Read the model definition and answer for the solid it produces. Units are mm, in the model's axes. Coordinates: 2 decimals unless noted, no trailing zeros. Write each loop counter-clockwise with the first axis right and the second up, starting at its lowest first coordinate (ties: lowest second). Pieces come first, ordered by that corner, then holes.
1) Find the intervals of material crossed by line 1 (Y direction, x = -254.5, z = 0.25); line 2 (Y direction, x = -270, z = 2.5); line 3 (Y direction, x = -81, z = -2), in increasing order.
2) The part is cut by section A-A (y = -1.5). Determine the outline of the cut face in (x, z), then the cut area to 3 significant figures.
3) Each of these flat-tipped pins is pushed along its axis until it touches: pin 1 Ø1.5 at (x, z) = (-178.5, 1) entering from +Y; pin 2 Ø5 at (x, y) = (-289, 0) entering from +Z; pin 3 Ø7.5 at (x, y) = (-275, 14.5) entering from +Z. Where does it stop, or does it pass through?
from build123d import *

# Parameters (mm, degrees)
BOSS_EXTRUDE1_DEPTH = 500.126
SKETCH2_W           = 12.7
SKETCH2_H           = 24.13
CUT_EXTRUDE1_DEPTH  = 505.455221633
SKETCH3_W           = 487.426
SKETCH3_H           = 14.75620072
BOSS_EXTRUDE2_DEPTH = 3.55599999
SKETCH4_W           = 3.55599999
SKETCH4_H           = 13.202768596
CUT_EXTRUDE2_DEPTH  = 501.46835993
DRAFT1_ANGLE        = 25
DRAFT2_ANGLE        = 25
FILLET1_R           = 0.76200009
FILLET2_R           = 1.98120009
FILLET3_R           = 2.54


with BuildPart() as part:
    # Sketch1 → Boss-Extrude1 (new body)
    with BuildSketch(Plane(origin=(-3.937, 0, 0), x_dir=(0, 0, -1), z_dir=(1, 0, 0))):
        with BuildLine():
            Line((2.311399989, 16.37657286), (2.311399989, -16.37657286))
            ThreePointArc((2.311399989, -16.37657286), (0.354826715, -15.481038557), (-1.770730805, -15.815950332))
            ThreePointArc((-1.770730805, -15.815950332), (-3.400639082, -15.955235788), (-4.710462095, -14.975253591))
            Line((-4.710462095, -14.975253591), (-5.7404, -15.627692517))
            ThreePointArc((-5.7404, -15.627692517), (-3.73586423, -17.127444277), (-1.241474216, -16.914283663))
            ThreePointArc((-1.241474216, -16.914283663), (0.188944014, -16.688900954), (1.505642365, -17.291560998))
            ThreePointArc((1.505642365, -17.291560998), (2.81343034, -17.487614789), (3.53059999, -16.37657286))
            Line((3.53059999, -16.37657286), (3.53059999, 16.37657286))
            ThreePointArc((3.53059999, 16.37657286), (2.81343034, 17.487614789), (1.505642365, 17.291560998))
            ThreePointArc((1.505642365, 17.291560998), (0.188944014, 16.688900954), (-1.241474216, 16.914283663))
            ThreePointArc((-1.241474216, 16.914283663), (-3.73586423, 17.127444277), (-5.7404, 15.627692517))
            Line((-5.7404, 15.627692517), (-4.710462095, 14.975253591))
            ThreePointArc((-4.710462095, 14.975253591), (-3.400639082, 15.955235788), (-1.770730805, 15.815950332))
            ThreePointArc((-1.770730805, 15.815950332), (0.354826715, 15.481038557), (2.311399989, 16.37657286))
        make_face()
    extrude(amount=-BOSS_EXTRUDE1_DEPTH)

    # Sketch2 → Cut-Extrude1 (cut, through all)
    with BuildSketch(Plane(origin=(0, 0, -3.53059999), x_dir=(-1, 0, 0), z_dir=(0, 0, -1))):
        with Locations((10.287, 0)):
            Rectangle(SKETCH2_W, SKETCH2_H)
    extrude(amount=-CUT_EXTRUDE1_DEPTH, mode=Mode.SUBTRACT)

    # Sketch3 → Boss-Extrude2 (add)
    with BuildSketch(Plane.XY.offset(-2.311399989)):
        with Locations((-260.35, 0)):
            Rectangle(SKETCH3_W, SKETCH3_H)
    extrude(amount=BOSS_EXTRUDE2_DEPTH)

    # Sketch4 → Cut-Extrude2 (cut, through all)
    with BuildSketch(Plane.ZY.offset(504.063)):
        with Locations((-1.752599995, 0)):
            Rectangle(SKETCH4_W, SKETCH4_H)
    extrude(amount=-CUT_EXTRUDE2_DEPTH, mode=Mode.SUBTRACT)

    # Draft1
    draft1_faces = [part.faces().sort_by_distance(p)[0] for p in [
        (-260.35, 7.37810036, -0.533399994),
        (-260.35, -7.37810036, -0.533399994),
    ]]
    draft(draft1_faces, Plane.XY.offset(1.244600001), DRAFT1_ANGLE)

    # Draft2
    draft2_faces = [part.faces().sort_by_distance(p)[0] for p in [
        (-260.35, 6.601384298, -1.752599995),
        (-260.35, -6.601384298, -1.752599995),
    ]]
    draft(draft2_faces, Plane(origin=(-3.937, -6.601384298, 0.0254), x_dir=(0, -1, 0), z_dir=(0, 0, -1)), DRAFT2_ANGLE)

    # Fillet1
    fillet1_edges = [part.edges().sort_by_distance(p)[0] for p in [
        (-260.35, -9.036290388, -2.311399989),
        (-260.35, 9.036290388, -2.311399989),
        (-260.35, 6.601384298, 0.0254),
        (-260.35, -6.601384298, 0.0254),
    ]]
    fillet(fillet1_edges, radius=FILLET1_R)

    # Fillet2
    fillet2_edges = [part.edges().sort_by_distance(p)[0] for p in [
        (-260.35, -7.37810036, 1.244600001),
        (-260.35, 7.37810036, 1.244600001),
        (-260.35, 8.259574326, -3.53059999),
        (-260.35, -8.259574326, -3.53059999),
    ]]
    fillet(fillet2_edges, radius=FILLET2_R)

    # Fillet3
    fillet3_edges = [part.edges().sort_by_distance(p)[0] for p in [
        (-16.637, 12.065, -2.92099999),
        (-16.637, -12.065, -2.92099999),
    ]]
    fillet(fillet3_edges, radius=FILLET3_R)


solid = part.part
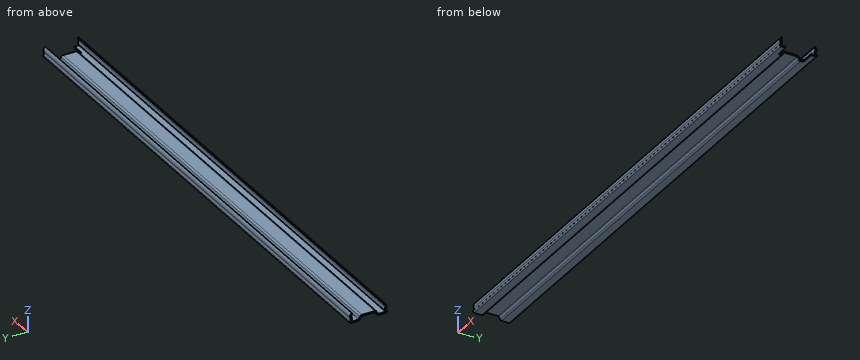
Reported:
1. line 1: y = -16.67 to -15.45, -7.83 to 7.83, 15.45 to 16.67
1. line 2: y = -17.25 to -16.03, 16.03 to 17.25
1. line 3: y = -17.56 to -16.13, -8.91 to -7.55, 7.55 to 8.91, 16.13 to 17.56
2. outline: (-504.06, 0.03) - (-16.64, 0.03) - (-16.64, 1.24) - (-504.06, 1.24) - close
2. area: 594 mm2
3. pin 1: stops at y = 17.11
3. pin 2: stops at z = 1.24
3. pin 3: stops at z = 5.74
